Part model, mm, in its own coordinate system. Face numbers are marked on the shaded views. A direction names the side the tool comes from. Round coordinates to 2 decimals unless told otherwise and drop trailing zeros. Loops run counter-clockwise (first coordinate to the right, second up) from the corner with the lowest first, then second, coordinate; pieces in that order, holes last.
1) Band-saw the part on C-C, the plane z = 15. Write the cut outline in (x, y), then the cut area to 3 significant figures.
2) Drop a flat-ended pin along its axis: P1, Ø6, axis at x = -45, z = 2, coming from the -Y side. Give the stop position or say it passes through.
3) Band-saw the part on A-A, the plane y = 98. Write the cut outline in (x, z).
4) 3-axis set-ups, long thin cutter, end or side, ignore diameter. For the marked faces 5 and 6: which of +Z, -Z, +X, -X, +Y, -Y reach the whole face in a straight line?
5) Probe line 1 (Z direction, x = -19.5, y = 99.5); line 2 (X direction, y = 50, z = 75.5); line 3 (Y direction, x = 22.5, z = 64.5). List the from-to ranges inside material, lowest first.
6) Mould opens along Z. For the marked faces 1, 2, 3 and 4 say: +Z half, -Z half, draft (parallel to the pull), parting line (faces both ways), or undercut.
7) Band-saw the part on B-B, the plane x = 57.5. Write the cut outline in (y, z).
from build123d import *

# Parameters (mm, degrees)
F0_W     = 150
F0_H     = 200
F1_DEPTH = 150
F2_T     = -12
F3_W     = 126
F3_H     = 12
F4_DEPTH = 140


with BuildPart() as f1:
    # F0 (on Front) → F1 (new body)
    with BuildSketch(Plane.XZ):
        Rectangle(F0_W, F0_H)
    extrude(amount=-F1_DEPTH)

    # F2
    f2_openings = [f1.faces().sort_by_distance(p)[0] for p in [
        (0, 0, 0),
    ]]
    offset(amount=F2_T, openings=f2_openings)

    # F3 (on face) → F4 (join)
    with BuildSketch(Plane.XZ):
        with Locations((0, 37.173926213)):
            Rectangle(F3_W, F3_H)
        with Locations((0, -40.3645330455)):
            Rectangle(F3_W, F3_H)
    extrude(amount=-F4_DEPTH)


solid = f1.part
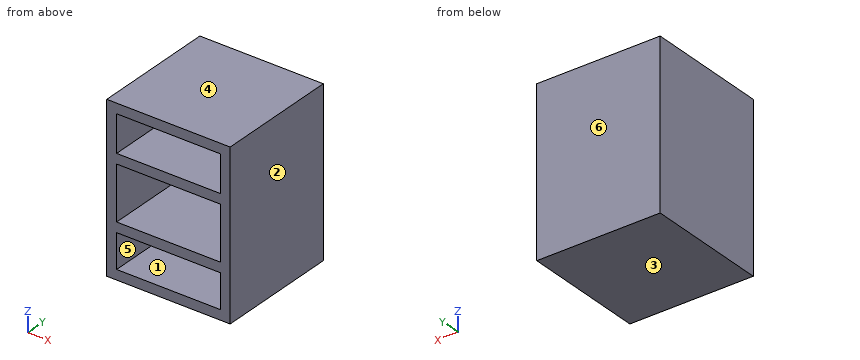
Reported:
1. outline: (-75, 0) - (-63, 0) - (-63, 138) - (63, 138) - (63, 0) - (75, 0) - (75, 150) - (-75, 150) - close
1. area: 5,110 mm2
2. P1: stops at y = 138
3. outline: (-75, -100) - (75, -100) - (75, 100) - (-75, 100) - close; hole (-63, -88) - (63, -88) - (63, -46.36) - (-63, -46.36) - close; hole (-63, -34.36) - (63, -34.36) - (63, 31.17) - (-63, 31.17) - close; hole (-63, 43.17) - (63, 43.17) - (63, 88) - (-63, 88) - close
4. face 5: -Y
4. face 6: +Z, -Z, +X, -X, +Y
5. line 1: z = -100 to -88, -46.36 to -34.36, 31.17 to 43.17, 88 to 100
5. line 2: x = -75 to -63, 63 to 75
5. line 3: y = 138 to 150
6. face 1: undercut
6. face 2: draft
6. face 3: -Z half
6. face 4: +Z half
7. outline: (0, -100) - (150, -100) - (150, 100) - (0, 100) - (0, 88) - (138, 88) - (138, 43.17) - (0, 43.17) - (0, 31.17) - (138, 31.17) - (138, -34.36) - (0, -34.36) - (0, -46.36) - (138, -46.36) - (138, -88) - (0, -88) - close
